Read the model definition and answer for the solid it produces. Units are mm, in the model's axes. Give positions to 0.01 mm unless a question says otherwise; leave off trailing zeros. Write each loop counter-clockwise with the first axis right and the second up, starting at its lowest first coordinate (ties: lowest second). Pieces come first, ordered by that corner, then holes. Notation, with made-up numbers: (75.25, 22) -> (129.25, 22) arc R19 ccw to (129.25, 27) -> close; hole circle Ø5 at (60.5, -20.5). An arc over 180 degrees is marked (long way). Use a Markdown table: item, result.
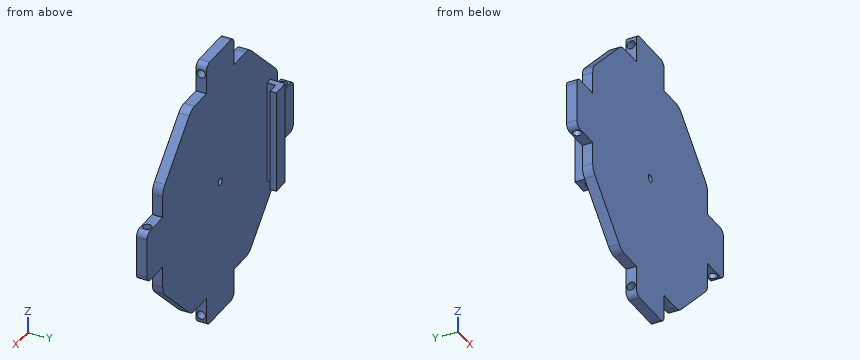
from build123d import *

# Parameters (mm, degrees)
SKETCH_1_W          = 14.3
SKETCH_1_H          = 25
SKETCH_1_W_2        = 25
SKETCH_1_H_2        = 14.3
EXTRUDE_1_DEPTH     = 5
FILLET_1_R          = 3
FILLET_2_R          = 7
FILLET_3_R          = 23
EXTRUDE_START       = -5
EXTRUDE_2_DEPTH     = 5
SKETCH_7_R          = 1.75
CUT_EXTRUDE_5_DEPTH = 94.895580301
SKETCH_9_W          = 3
SKETCH_9_H          = 50
EXTRUDE_3_DEPTH     = 7
SKETCH_10_W         = 50
SKETCH_10_H         = 3
EXTRUDE_4_DEPTH     = 5
SKETCH_11_R         = 2
CUT_EXTRUDE_6_DEPTH = 104.678011169
SKETCH_12_R         = 2
CUT_EXTRUDE_7_DEPTH = 104.678011169


with BuildPart() as part:
    # 스케치1 → 보스-돌출1 (new body)
    with BuildSketch(Plane(origin=(0, 0, 0), x_dir=(1, 0, 0), z_dir=(0, 1, 0))):
        Polygon((-26, 52), (-39, 39), (-26, 39), (26, 39), (39, 39), (26, 52), (12.5, 52), (-12.5, 52), align=None)
        Polygon((-26, 39), (-39, 39), (-39, 26), align=None)
        Polygon((-39, 26), (-39, 39), (-52, 26), (-52, 12.5), (-52, -12.5), (-52, -26), (-39, -39), (-39, -26), align=None)
        with Locations((-59.15, 0)):
            Rectangle(SKETCH_1_W, SKETCH_1_H)
        with Locations((0, 59.15)):
            Rectangle(SKETCH_1_W_2, SKETCH_1_H_2)
        Polygon((39, 39), (26, 39), (39, 26), align=None)
        Polygon((52, 26), (39, 39), (39, 26), (39, -26), (39, -39), (52, -26), (52, -12.5), (52, 12.5), align=None)
        with Locations((59.15, 0)):
            Rectangle(SKETCH_1_W, SKETCH_1_H)
        Polygon((39, -39), (39, -26), (26, -39), align=None)
        Polygon((-26, -39), (-39, -39), (-26, -52), (-12.5, -52), (12.5, -52), (26, -52), (39, -39), (26, -39), align=None)
        Polygon((-26, -39), (-39, -26), (-39, -39), align=None)
        with Locations((0, -59.15)):
            Rectangle(SKETCH_1_W_2, SKETCH_1_H_2)
    extrude(amount=EXTRUDE_1_DEPTH)

    # 필렛1
    fillet_1_edges = [part.edges().sort_by_distance(p)[0] for p in [
        (12.5, 2.5, 66.3),
        (-12.5, 2.5, 66.3),
        (-66.3, 2.5, 12.5),
        (-66.3, 2.5, -12.5),
        (-12.5, 2.5, -66.3),
        (12.5, 2.5, -66.3),
        (66.3, 2.5, -12.5),
        (66.3, 2.5, 12.5),
    ]]
    fillet(fillet_1_edges, radius=FILLET_1_R)

    # 필렛2
    fillet_2_edges = [part.edges().sort_by_distance(p)[0] for p in [
        (-26, 2.5, 52),
        (-52, 2.5, 26),
        (-52, 2.5, -26),
        (-26, 2.5, -52),
        (26, 2.5, -52),
        (52, 2.5, -26),
        (52, 2.5, 26),
        (26, 2.5, 52),
    ]]
    fillet(fillet_2_edges, radius=FILLET_2_R)

    # 필렛3
    # the kernel refuses this fillet: 23 mm, written as the material it adds along each edge
    with BuildSketch(Plane(origin=(-39, 0, 26), x_dir=(0, 0, -1), z_dir=(0, 1, 0))) as fillet_3_piece_1:
        with BuildLine():
            CenterArc((FILLET_3_R * 0.414213562373, -FILLET_3_R), FILLET_3_R, 90, 45)
            Line((-FILLET_3_R * 0.292893218813, -FILLET_3_R * 0.292893218813), (0, 0))
            Line((0, 0), (FILLET_3_R * 0.414213562373, 0))
        make_face()
    extrude(amount=5)
    with BuildSketch(Plane(origin=(-26, 0, 39), x_dir=(1, 0, 0), z_dir=(0, 1, 0)), Plane(origin=(26, 0, 39), x_dir=(0.7071067811865479, 0, -0.7071067811865471), z_dir=(0, 1, 0)), Plane(origin=(39, 0, 26), x_dir=(0, 0, -1), z_dir=(0, 1, 0)), Plane(origin=(39, 0, -26), x_dir=(-0.7071067811865476, 0, -0.7071067811865476), z_dir=(0, 1, 0)), Plane(origin=(26, 0, -39), x_dir=(-1, 0, 0), z_dir=(0, 1, 0)), Plane(origin=(-26, 0, -39), x_dir=(-0.7071067811865471, 0, 0.7071067811865479), z_dir=(0, 1, 0)), Plane(origin=(-39, 0, -26), x_dir=(0, 0, 1), z_dir=(0, 1, 0))) as fillet_3_piece_2:
        with BuildLine():
            CenterArc((FILLET_3_R * 0.414213562373, FILLET_3_R), FILLET_3_R, 225, 45)
            Line((-FILLET_3_R * 0.292893218813, FILLET_3_R * 0.292893218813), (0, 0))
            Line((0, 0), (FILLET_3_R * 0.414213562373, 0))
        make_face()
    extrude(amount=5)

    # 스케치6 → 보스-돌출2 (add)
    with BuildSketch(Plane(origin=(0, 5, 0), x_dir=(1, 0, 0), z_dir=(0, 1, 0)).offset(EXTRUDE_START)):
        with BuildLine():
            Line((16.473088065, 39), (-16.473088065, 39))
            ThreePointArc((-16.473088065, 39), (-25.120040329, 37.312677367), (-32.4982797, 32.4982797))
            ThreePointArc((-32.4982797, 32.4982797), (-37.312677367, 25.120040329), (-39, 16.473088065))
            Line((-39, 16.473088065), (-39, -16.473088065))
            ThreePointArc((-39, -16.473088065), (-37.312677367, -25.120040329), (-32.4982797, -32.4982797))
            ThreePointArc((-32.4982797, -32.4982797), (-25.120040329, -37.312677367), (-16.473088065, -39))
            Line((-16.473088065, -39), (16.473088065, -39))
            ThreePointArc((16.473088065, -39), (25.120040329, -37.312677367), (32.4982797, -32.4982797))
            ThreePointArc((32.4982797, -32.4982797), (37.312677367, -25.120040329), (39, -16.473088065))
            Line((39, -16.473088065), (39, 16.473088065))
            ThreePointArc((39, 16.473088065), (37.312677367, 25.120040329), (32.4982797, 32.4982797))
            ThreePointArc((32.4982797, 32.4982797), (25.120040329, 37.312677367), (16.473088065, 39))
        make_face()
    extrude(amount=EXTRUDE_2_DEPTH)

    # 스케치7 → 컷-돌출5 (cut, through all)
    with BuildSketch(Plane(origin=(0, 5, 0), x_dir=(1, 0, 0), z_dir=(0, 1, 0))):
        with Locations(Location((0, 0, 0), (0, 0, 270))):
            Circle(SKETCH_7_R)
    extrude(amount=-CUT_EXTRUDE_5_DEPTH, mode=Mode.SUBTRACT)

    # 스케치9 → 보스-돌출3 (add)
    with BuildSketch(Plane(origin=(0, 5, 0), x_dir=(1, 0, 0), z_dir=(0, 1, 0))):
        with Locations((-44, 0)):
            Rectangle(SKETCH_9_W, SKETCH_9_H)
    extrude(amount=EXTRUDE_3_DEPTH)

    # 스케치10 → 보스-돌출4 (add)
    with BuildSketch(Plane(origin=(-42.5, 0, 0), x_dir=(0, 0, -1), z_dir=(1, 0, 0))):
        with Locations((0, 10.5)):
            Rectangle(SKETCH_10_W, SKETCH_10_H)
    extrude(amount=EXTRUDE_4_DEPTH)

    # 스케치11 → 컷-돌출6 (cut, through all)
    with BuildSketch(Plane.XY.offset(12.5)):
        with Locations(Location((-61.3, 2.5, 0), (0, 0, 180))):
            Circle(SKETCH_11_R)
        with Locations((61.3, 2.5)):
            Circle(SKETCH_11_R)
    extrude(amount=-CUT_EXTRUDE_6_DEPTH, mode=Mode.SUBTRACT)

    # 스케치12 → 컷-돌출7 (cut, through all)
    with BuildSketch(Plane.ZY.offset(12.5)):
        with Locations(Location((-61.3, 2.5, 0), (0, 0, 180))):
            Circle(SKETCH_12_R)
        with Locations((61.3, 2.5)):
            Circle(SKETCH_12_R)
    extrude(amount=-CUT_EXTRUDE_7_DEPTH, mode=Mode.SUBTRACT)


solid = part.part
Item 1: A cutting plane is placed at D-D (z = -18). Give the vertices of the cut face in (x, y).
Return value:
| item | result |
|---|---|
| outline | (-52, 0) -> (52, 0) -> (52, 5) -> (-42.5, 5) -> (-42.5, 9) -> (-37.5, 9) -> (-37.5, 12) -> (-45.5, 12) -> (-45.5, 5) -> (-52, 5) -> close |
Item 2: A cutting plane is placed at B-B (x = 0). Give the vertices of the cut face in (y, z).
Return value:
| item | result |
|---|---|
| outline | (0, -66.3) -> (5, -66.3) -> (5, -1.75) -> (0, -1.75) -> close; (0, 1.75) -> (5, 1.75) -> (5, 66.3) -> (0, 66.3) -> close; hole circle Ø4 at (2.5, -61.3); hole circle Ø4 at (2.5, 61.3) |
Item 3: A cutting plane is placed at C-C (x = -61.3). Give the vertices of the cut face in (y, z).
Return value:
| item | result |
|---|---|
| outline | (0, -12.5) -> (0.5, -12.5) -> (0.5, 12.5) -> (0, 12.5) -> close; (4.5, -12.5) -> (5, -12.5) -> (5, 12.5) -> (4.5, 12.5) -> close |
Item 4: A cutting plane is placed at A-A (z = 0). Give the vertices of the cut face in (x, y).
Return value:
| item | result |
|---|---|
| outline | (-66.3, 0) -> (-1.75, 0) -> (-1.75, 5) -> (-42.5, 5) -> (-42.5, 9) -> (-37.5, 9) -> (-37.5, 12) -> (-45.5, 12) -> (-45.5, 5) -> (-66.3, 5) -> close; (1.75, 0) -> (66.3, 0) -> (66.3, 5) -> (1.75, 5) -> close; hole circle Ø4 at (-61.3, 2.5); hole circle Ø4 at (61.3, 2.5) |
Item 5: Each of these flat-tipped pins is pushed along its axis until it touches: P1, Ø4, axis at y = 3.5, z = 15.5, coming from the -X side; P2, Ø1.5, axis at x = -57, y = 2, coming from the +Z side; P3, Ø5.5, axis at y = 3, z = 59, coming from the +X side. Where does it stop, or does it pass through?
Return value:
| item | result |
|---|---|
| P1 | x = -52 |
| P2 | z = 12.5 |
| P3 | x = 12.5 |
Item 6: Straight lines are drawn through the part: line 1 along Y through (x, z) = (-38, 7.5); line 2 along Y through (x, z) = (-3, 61.3); line 3 along X through (y, z) = (4, -2). For each, find the intervals that lie inside material, in ascending order. Write a range as [from, to].
Return value:
| item | result |
|---|---|
| line 1 | [0, 5], [9, 12] |
| line 2 | [0, 0.5], [4.5, 5] |
| line 3 | [-66.3, -62.62], [-59.98, 59.98], [62.62, 66.3] |
